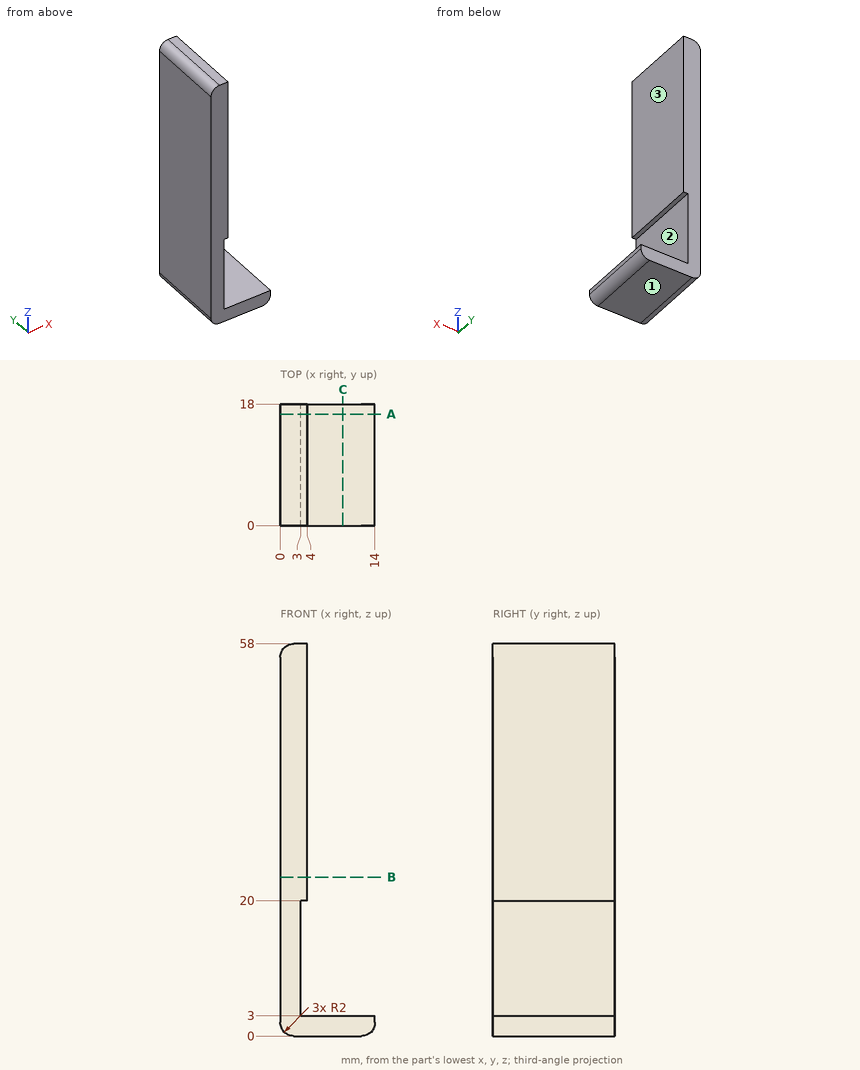
The figure shows three views and two pictorial views of one solid part (mm, origin at its lowest corner). Answer the questions. Give positions to 0.01 mm unless a question says otherwise; leave off trailing zeros. Loops run counter-clockwise (first coordinate to the right, second up) from the corner with the lowest first, then second, coordinate; pieces in that order, holes last. Notation, with made-up numbers: (76.5, 37) -> (122.5, 37) arc R15 cw to (122.5, 46) -> close; hole circle Ø3 at (-28.75, 14). An arc over 180 degrees is marked (long way). Use a Markdown table: item, result. Add a question column.
1. Determine the mould class of the marked faces 1, 2 and 3 for opening direction Z: released by +Z, released by -Z, zero draft, split by the parting line, or undercut.
2. Find the intervals of material crossed by probe 1 along Z at (x, y) = (3.75, 17); probe 2 along X at (y, z) = (15.75, 48); probe 3 along X at (y, z) = (16, 4.5), in increasing order.
3. Section B-B on z = 23.5 is taken. Determine the outline of the cut face in (x, y).
4. Section A-A on y = 16.5 is taken. Determine the outline of the cut face in (x, z).
5. Flat-ended cylindrical pins translate along their axes: pin 1 Ø9 at (y, z) = (12.5, 42.5) entering from +X; pin 2 Ø8.5 at (y, z) = (5.5, 12.5) entering from +X. Find the tip coordinate at first contact, or state that the pin passes through.
6. Section C-C on x = 9.25 is taken. Determine the outline of the cut face in (y, z), and give its area (3 significant figures).
Results below:
| question | item | result |
|---|---|---|
| 1 | face 1 | released by -Z |
| 1 | face 2 | undercut |
| 1 | face 3 | zero draft |
| 2 | probe 1 | z = 0 to 3, 20 to 58 |
| 2 | probe 2 | x = 0 to 4 |
| 2 | probe 3 | x = 0 to 3 |
| 3 | outline | (0, 0) -> (4, 0) -> (4, 18) -> (0, 18) -> close |
| 4 | outline | (0, 2) arc R2 ccw to (2, 0) -> (12, 0) arc R2 ccw to (14, 2) -> (14, 3) -> (3, 3) -> (3, 20) -> (4, 20) -> (4, 58) -> (2, 58) arc R2 ccw to (0, 56) -> close |
| 5 | pin 1 | stops at x = 4 |
| 5 | pin 2 | stops at x = 3 |
| 6 | outline | (0, 0) -> (18, 0) -> (18, 3) -> (0, 3) -> close |
| 6 | area | 54.0 mm^2 |
